```python
from build123d import *

# Parameters (mm, degrees)
F0_W     = 140
F0_H     = 70
F1_DEPTH = 10
F2_R     = 16
F4_DEPTH = 25


with BuildPart() as f1:
    # F0 (on Front) → F1 (new body)
    with BuildSketch(Plane.XZ):
        with Locations((70, 35)):
            Rectangle(F0_W, F0_H)
    extrude(amount=F1_DEPTH)

    # F2
    f2_edges = [f1.edges().sort_by_distance(p)[0] for p in [
        (0, -5, 0),
        (140, -5, 0),
        (140, -5, 70),
        (0, -5, 70),
    ]]
    fillet(f2_edges, radius=F2_R)

    # F3 (on face) → F4 (join)
    with BuildSketch(Plane(origin=(0, 0, 0), x_dir=(-1, 0, 0), z_dir=(0, 1, 0))):
        with BuildLine():
            ThreePointArc((-105, 47.5), (-96.1611652352, 43.8388347648), (-92.5, 35))
            Line((-92.5, 35), (-87.5, 35))
            ThreePointArc((-87.5, 35), (-87.5449306601, 36.2532175939), (-87.6794919243, 37.5))
            ThreePointArc((-87.6794919243, 37.5), (-93.5435607626, 48.2287565553), (-105, 52.5))
            Line((-105, 52.5), (-105, 47.5))
        make_face()
        with BuildLine():
            ThreePointArc((-117.5, 35), (-113.8388347648, 43.8388347648), (-105, 47.5))
            Line((-105, 47.5), (-105, 52.5))
            ThreePointArc((-105, 52.5), (-117.3743686708, 47.3743686708), (-122.5, 35))
            Line((-122.5, 35), (-117.5, 35))
        make_face()
        with BuildLine():
            Line((-105, 17.5), (-105, 22.5))
            ThreePointArc((-105, 22.5), (-113.8388347648, 26.1611652352), (-117.5, 35))
            Line((-117.5, 35), (-122.5, 35))
            ThreePointArc((-122.5, 35), (-117.3743686708, 22.6256313292), (-105, 17.5))
        make_face()
        with BuildLine():
            Line((-87.5, 35), (-92.5, 35))
            ThreePointArc((-92.5, 35), (-96.1611652352, 26.1611652352), (-105, 22.5))
            Line((-105, 22.5), (-105, 17.5))
            ThreePointArc((-105, 17.5), (-93.5435607626, 21.7712434447), (-87.6794919243, 32.5))
            ThreePointArc((-87.6794919243, 32.5), (-87.5449306601, 33.7467824061), (-87.5, 35))
        make_face()
        with BuildLine():
            ThreePointArc((-52.3205080757, 37.5), (-52.4550693399, 36.2532175939), (-52.5, 35))
            Line((-52.5, 35), (-47.5, 35))
            ThreePointArc((-47.5, 35), (-35, 47.5), (-22.5, 35))
            Line((-22.5, 35), (-17.5, 35))
            ThreePointArc((-17.5, 35), (-33.7467824061, 52.4550693399), (-52.3205080757, 37.5))
        make_face()
        with BuildLine():
            Line((-47.5, 35), (-52.5, 35))
            ThreePointArc((-52.5, 35), (-52.4550693399, 33.7467824061), (-52.3205080757, 32.5))
            ThreePointArc((-52.3205080757, 32.5), (-33.7467824061, 17.5449306601), (-17.5, 35))
            Line((-17.5, 35), (-22.5, 35))
            ThreePointArc((-22.5, 35), (-35, 22.5), (-47.5, 35))
        make_face()
        with BuildLine():
            ThreePointArc((-87.6794919243, 37.5), (-87.5449306601, 36.2532175939), (-87.5, 35))
            Line((-87.5, 35), (-52.5, 35))
            ThreePointArc((-52.5, 35), (-52.4550693399, 36.2532175939), (-52.3205080757, 37.5))
            Line((-52.3205080757, 37.5), (-70, 37.5))
            Line((-70, 37.5), (-87.6794919243, 37.5))
        make_face()
        with BuildLine():
            Line((-52.5, 35), (-87.5, 35))
            ThreePointArc((-87.5, 35), (-87.5449306601, 33.7467824061), (-87.6794919243, 32.5))
            Line((-87.6794919243, 32.5), (-70, 32.5))
            Line((-70, 32.5), (-52.3205080757, 32.5))
            ThreePointArc((-52.3205080757, 32.5), (-52.4550693399, 33.7467824061), (-52.5, 35))
        make_face()
    extrude(amount=F4_DEPTH)


solid = f1.part
```
The model under review builds one solid part; all positions refer to its coordinate system, in mm. A direction names the side the tool comes from. Round coordinates to 2 decimals unless told otherwise and drop trailing zeros. Order: outer loops, then holes, each group sorted by start corner. A loop starts at its lowest first (then second) coordinate and runs counter-clockwise, first axis right, second up. Notation, with made-up numbers: (-26, 74) - (-8, 74) arc R33 ccw to (-8, 108) - close; hole circle Ø8 at (84.25, 3.25). An arc over 180 degrees is marked (long way). Answer in a Markdown table with one row per item.
(1) Take a section at D-D on z = 49.5. Write out the cut boundary in (x, y).
Result set:
| item | result |
|---|---|
| outline | (0, -10) - (140, -10) - (140, 0) - (114.8, 0) - (114.8, 25) - (95.2, 25) - (95.2, 0) - (44.8, 0) - (44.8, 25) - (25.2, 25) - (25.2, 0) - (0, 0) - close |
(2) Take a section at A-A on y = 16.5. Write out the cut boundary in (x, z).
Result set:
| item | result |
|---|---|
| outline | (52.32, 32.5) - (87.68, 32.5) arc R17.5 ccw (long way) to (87.68, 37.5) - (52.32, 37.5) arc R17.5 ccw (long way) to start; hole circle Ø25 at (35, 35); hole circle Ø25 at (105, 35) |
(3) For line 1 (X direction, y = 5, z = 35); line 2 (Z direction, x = 35, y = 9.5); line 3 (X direction, y = 6.5, z = 28.5), list the stretches that pass through material, from the lowest coordinate up. Write a range as from..to.
Result set:
| item | result |
|---|---|
| line 1 | x = 17.5..22.5, 47.5..92.5, 117.5..122.5 |
| line 2 | z = 17.5..22.5, 47.5..52.5 |
| line 3 | x = 18.75..24.32, 45.68..51.25, 88.75..94.32, 115.68..121.25 |
(4) Machinability: for faces 5 (the face through (69, 0, 43)), 6 (the face through (70, 12, 32.5)), 7 (the face through (4.563, -5.07, 65.189)), which of the approach directions +Z, -Z, +X, -X, +Y, -Y give a long, thin tool a straight path to every point of the face, cutting with its end or side? Answer none if there is none.
Result set:
| item | result |
|---|---|
| face 5 | +Y |
| face 6 | -Z, +Y |
| face 7 | +Z, -X, +Y, -Y |
(5) Take a section at C-C on y = -3. Write out the cut boundary in (x, z), plus the area to 3 significant figures.
Result set:
| item | result |
|---|---|
| outline | (0, 16) arc R16 ccw to (16, 0) - (124, 0) arc R16 ccw to (140, 16) - (140, 54) arc R16 ccw to (124, 70) - (16, 70) arc R16 ccw to (0, 54) - close |
| area | 9,580 mm2 |
(6) Clearance check with flat-ended pins moving along their axes: P1, Ø12, axis at y = 6.5, z = 18, coming from the +X side; P2, Ø8, axis at x = 92, y = 16.5, coming from the +Z side; P3, Ø3, axis at x = 101, y = 9, coming from the -Z side. State where each tip first meets the part, or that it passes through.
Result set:
| item | result |
|---|---|
| P1 | stops at x = 118.61 |
| P2 | stops at z = 50.01 |
| P3 | stops at z = 17.68 |
(7) Mouldability with a two-part tool opening along Z and no side actions: class faces 1 (the face through (105, 0, 35)), 2 (the face through (35, 0, 35)), 3 (the face through (140, -5, 35)), 4 (the face through (70, 12, 37.5)) as released by +Z, released by -Z, zero draft, split by the parting line, or undercut.
Result set:
| item | result |
|---|---|
| face 1 | undercut |
| face 2 | undercut |
| face 3 | zero draft |
| face 4 | released by +Z |
(8) Take a section at B-B on x = 63.5. Write out the cut boundary in (y, z).
Result set:
| item | result |
|---|---|
| outline | (-10, 0) - (0, 0) - (0, 32.5) - (25, 32.5) - (25, 37.5) - (0, 37.5) - (0, 70) - (-10, 70) - close |
